Verification items for this drawing (mm, ordinates from the low corner). A direction names the side the tool comes from. Give positions to 0.01 mm unless a question says otherwise; leave off trailing zeros. Order: outer loops, then holes, each group sorted by start corner. A loop starts at its lowest first (then second) coordinate and runs counter-clockwise, first axis right, second up. Notation, with made-up numbers: M 70,69 L 119,69 A9 cw 119,83 Z; hole C 32,-3 d5. An arc over 180 degrees is marked long. Answer as a JSON object with one key per item and string values.
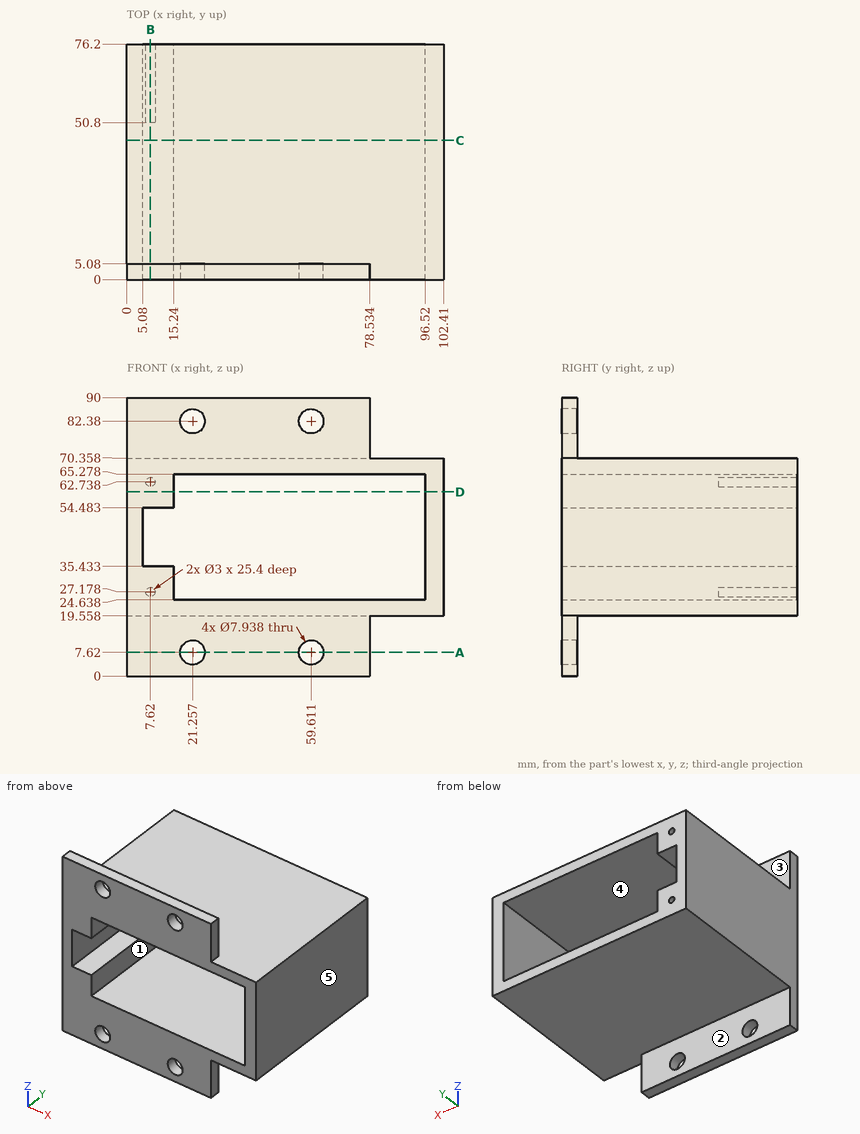
Q1. Section check A-A on z = 7.62. Record the cut outline in (x, y) (1 decimal), then the cut area to 3 significant figures.
Resolved:
{"outline": "M 0,0 L 17.3,0 L 17.3,5.1 L 0,5.1 Z; M 25.2,0 L 55.6,0 L 55.6,5.1 L 25.2,5.1 Z; M 63.6,0 L 78.5,0 L 78.5,5.1 L 63.6,5.1 Z", "area": "318 mm²"}
Q2. Gauge pin test, flat ends, axial feed: pin 1 Ø5 at (x, z) = (59.611, 82.38) entering from -Y (1 decimal); pin 2 Ø2.5 at (x, z) = (7, 62.5) entering from +Y; pin 3 Ø5 at (x, y) = (9, 40) entering from -Z; pin 4 Ø3 at (x, y) = (47.5, 37.5) entering from +Z. Record the tip position at first contact, or that the pin passes through.
Resolved:
{"pin 1": "passes through", "pin 2": "stops at y = 76.2", "pin 3": "stops at z = 19.56", "pin 4": "stops at z = 70.36"}
Q3. Material ranges on L1, parallel to X at y = 2.1, z = 7.62 (1 decimal); L2, parallel to Z at x = 7.62, y = 64; L3, parallel to X at y = 3, z = 82 (1 decimal), recorded low to high.
Resolved:
{"L1": "x = 0 to 17.3, 25.2 to 55.6, 63.6 to 78.5", "L2": "z = 19.56 to 25.68, 28.68 to 35.43, 54.48 to 61.24, 64.24 to 70.36", "L3": "x = 0 to 17.3, 25.2 to 55.7, 63.6 to 78.5"}
Q4. Release check for a two-part mould opening along Z. For the marked faces 4 and 5 record: +Z half, -Z half, draft (parallel to the pull), parting line (faces both ways), or undercut.
Resolved:
{"face 4": "undercut", "face 5": "draft"}
Q5. Section check B-B on x = 7.62. Record the cut outline in (y, z), then the cut area to 3 significant figures.
Resolved:
{"outline": "M 0,0 L 5.08,0 L 5.08,19.56 L 76.2,19.56 L 76.2,25.68 L 50.8,25.68 L 50.8,28.68 L 76.2,28.68 L 76.2,35.43 L 0,35.43 Z; M 0,54.48 L 76.2,54.48 L 76.2,61.24 L 50.8,61.24 L 50.8,64.24 L 76.2,64.24 L 76.2,70.36 L 5.08,70.36 L 5.08,90 L 0,90 Z", "area": "2,470 mm²"}
Q6. Section check C-C on y = 45. Record the cut outline in (x, z).
Resolved:
{"outline": "M 0,19.56 L 102.41,19.56 L 102.41,70.36 L 0,70.36 Z; hole M 5.08,35.43 L 15.24,35.43 L 15.24,24.64 L 96.52,24.64 L 96.52,65.28 L 15.24,65.28 L 15.24,54.48 L 5.08,54.48 Z"}
Q7. Tool access check on the marked faces 1, 2 and 3. Record the directions out of +Z, -Z, +X, -X, +Y, -Y that give a thin tool (end or side, any length) a straight path to the whole face; none if there is none.
Resolved:
{"face 1": "+Y, -Y", "face 2": "-Z, +X, -X, +Y", "face 3": "+Z, +X, -X, +Y"}
Q8. Section check D-D on z = 59.5. Record the cut outline in (x, y).
Resolved:
{"outline": "M 0,0 L 15.24,0 L 15.24,76.2 L 0,76.2 Z; M 96.52,0 L 102.41,0 L 102.41,76.2 L 96.52,76.2 Z"}
